Can you work these out from the model? Positions are in its coordinate system, mm. Face numbers are marked on the shaded views. Coordinates: 2 decimals unless noted, no trailing zeros. Write each loop counter-clockwise with the first axis right and the second up, starting at its lowest first coordinate (ties: lowest second). Pieces come first, ordered by that corner, then holes. Notation, with made-up numbers: (79, 38.25) - (130, 38.25) arc R29 cw to (130, 71.25) - close; hole circle Ø4 at (73.5, 87). An arc over 180 degrees is marked (long way). Write each question's results on one line, items separated by ' | '. Start each with the question number.
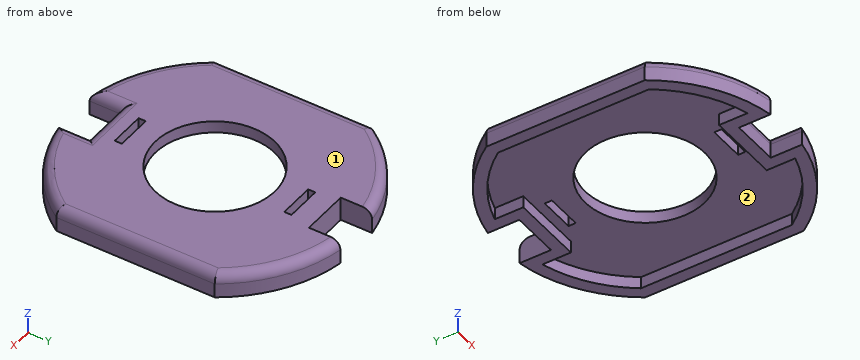
```python
from build123d import *

# Parameters (mm, degrees)
BOSS_EXTRUDE1_DEPTH = 1
FILLET1_R           = 0.4
SHELL1_DEPTH        = 0.5
SKETCH3_R           = 2.5
CUT_EXTRUDE1_DEPTH  = 1
CUT_EXTRUDE2_REACH  = 9.81
SKETCH4_W           = 1.5
SKETCH4_H           = 0.3


# Read off the part's stored shape, not the designer's step: Shell1
with BuildPart() as part:
    # Sketch2 → Boss-Extrude1 (new body)
    with BuildSketch(Plane.XY):
        with BuildLine():
            Line((-5, -3.31662479), (-5, 3.31662479))
            ThreePointArc((-5, 3.31662479), (-3.269448205, 5.030974899), (-1, 5.916079783))
            Line((-1, 5.916079783), (-1, 4.6))
            Line((-1, 4.6), (1, 4.6))
            Line((1, 4.6), (1, 5.916079783))
            ThreePointArc((1, 5.916079783), (3.269448205, 5.030974899), (5, 3.31662479))
            Line((5, 3.31662479), (5, -3.31662479))
            ThreePointArc((5, -3.31662479), (3.269448205, -5.030974899), (1, -5.916079783))
            Line((1, -5.916079783), (1, -4.6))
            Line((1, -4.6), (-1, -4.6))
            Line((-1, -4.6), (-1, -5.916079783))
            ThreePointArc((-1, -5.916079783), (-3.269448205, -5.030974899), (-5, -3.31662479))
        make_face()
    extrude(amount=BOSS_EXTRUDE1_DEPTH)

    # Fillet1
    fillet1_edges = [part.edges().sort_by_distance(p)[0] for p in [
        (3.269448205, 5.030974899, 1),
        (5, 0, 1),
        (3.269448205, -5.030974899, 1),
        (1, -5.258039892, 1),
        (0, -4.6, 1),
        (-1, -5.258039892, 1),
        (-3.269448205, -5.030974899, 1),
        (-5, 0, 1),
        (-3.269448205, 5.030974899, 1),
    ]]
    fillet(fillet1_edges, radius=FILLET1_R)

    # Shell1 outline → Shell1 (cut)
    with BuildSketch(Plane.XY):
        with BuildLine():
            ThreePointArc((1.5, -5.291502622), (3.183300133, -4.485153316), (4.5, -3.16227766))
            Line((4.5, -3.16227766), (4.5, 3.16227766))
            ThreePointArc((4.5, 3.16227766), (3.183300133, 4.485153316), (1.5, 5.291502622))
            Line((1.5, 5.291502622), (1.5, 4.1))
            Line((1.5, 4.1), (-1.5, 4.1))
            Line((-1.5, 4.1), (-1.5, 5.291502622))
            ThreePointArc((-1.5, 5.291502622), (-3.183300133, 4.485153316), (-4.5, 3.16227766))
            Line((-4.5, 3.16227766), (-4.5, -3.16227766))
            ThreePointArc((-4.5, -3.16227766), (-3.183300133, -4.485153316), (-1.5, -5.291502622))
            Line((-1.5, -5.291502622), (-1.5, -4.1))
            Line((-1.5, -4.1), (1.5, -4.1))
            Line((1.5, -4.1), (1.5, -5.291502622))
        make_face()
    extrude(amount=SHELL1_DEPTH, mode=Mode.SUBTRACT)

    # Sketch3 → Cut-Extrude1 (cut)
    with BuildSketch(Plane.XY.offset(1)):
        Circle(SKETCH3_R)
    extrude(amount=-CUT_EXTRUDE1_DEPTH, mode=Mode.SUBTRACT)

    # Sketch4 → Cut-Extrude2 (cut, up to next)
    with BuildSketch(Plane.XY.offset(1), mode=Mode.PRIVATE) as cut_extrude2_sk1:
        with Locations((0, 3.55)):
            Rectangle(SKETCH4_W, SKETCH4_H)
    cut_extrude2_tool1 = extrude(cut_extrude2_sk1.sketch, amount=-CUT_EXTRUDE2_REACH, mode=Mode.PRIVATE) & part.part
    # Sketch4 → Cut-Extrude2 (cut, up to next)
    with BuildSketch(Plane.XY.offset(1), mode=Mode.PRIVATE) as cut_extrude2_sk2:
        with Locations((0, -3.55)):
            Rectangle(SKETCH4_W, SKETCH4_H)
    cut_extrude2_tool2 = extrude(cut_extrude2_sk2.sketch, amount=-CUT_EXTRUDE2_REACH, mode=Mode.PRIVATE) & part.part
    add(cut_extrude2_tool1.solids().sort_by_distance((0, 3.55, 1))[0], mode=Mode.SUBTRACT)
    add(cut_extrude2_tool2.solids().sort_by_distance((0, -3.55, 1))[0], mode=Mode.SUBTRACT)


solid = part.part
```
Q1. I'm going to push flat-ended pins straight in: pin 1 Ø0.6 at (x, z) = (0.5, 0) entering from +Y; pin 2 Ø0.6 at (x, z) = (0.5, 1) entering from -Y. Where does each tip first touch, or does it pass through?
Q2. I need wall thicknesses on line 1 along X through (y, z) = (-2.25, 0.45); line 2 along X through (y, z) = (-4.75, 0.4); line 3 along Y through (x, z) = (0, 0.75). Which ranges of each line are inside material? Lowest first, please. Write a range as from..to.
Q3. If we section it at B-B (z = 0.15): Please give me the cut outline in (x, y), then the cut area to 3 significant figures.
Q4. If we section it at D-D (y = 2): Please give me the cut outline in (x, z), then the cut area to 3 significant figures.
Q5. Thinking about a two-plate mould opening in X: for the marked faces 1 and 2, which applies, pulls with the +X half, pulls with the -X half, needs draft (parallel to the pull), parting line crosses it, or undercut?
Q6. If we section it at A-A (y = 0): Please give me the cut outline in (x, z).
Q7. If we section it at C-C (x = 0): Please give me the cut outline in (y, z).
Answer list:
1) pin 1: stops at y = 4.6 | pin 2: stops at y = -4.59
2) line 1: x = -5..-4.5, 4.5..5 | line 2: x = -3.67..-2.77, -1.5..-1, 1..1.5, 2.77..3.67 | line 3: y = -4.57..-3.7, -3.4..-2.5, 2.5..3.4, 3.7..4.6
3) outline: (-5, -3.32) arc R6 ccw to (-1, -5.92) - (-1, -4.6) - (1, -4.6) - (1, -5.92) arc R6 ccw to (5, -3.32) - (5, 3.32) arc R6 ccw to (1, 5.92) - (1, 4.6) - (-1, 4.6) - (-1, 5.92) arc R6 ccw to (-5, 3.32) - close; hole (-4.5, -3.16) arc R5.5 ccw to (-1.5, -5.29) - (-1.5, -4.1) - (1.5, -4.1) - (1.5, -5.29) arc R5.5 ccw to (4.5, -3.16) - (4.5, 3.16) arc R5.5 ccw to (1.5, 5.29) - (1.5, 4.1) - (-1.5, 4.1) - (-1.5, 5.29) arc R5.5 ccw to (-4.5, 3.16) - close | area: 20.2 mm2
4) outline: (-5, 0) - (-4.5, 0) - (-4.5, 0.5) - (-1.5, 0.5) - (-1.5, 1) - (-4.6, 1) arc R0.4 ccw to (-5, 0.6) - close; (1.5, 0.5) - (4.5, 0.5) - (4.5, 0) - (5, 0) - (5, 0.6) arc R0.4 ccw to (4.6, 1) - (1.5, 1) - close | area: 3.93 mm2
5) face 1: needs draft | face 2: undercut
6) outline: (-5, 0) - (-4.5, 0) - (-4.5, 0.5) - (-2.5, 0.5) - (-2.5, 1) - (-4.6, 1) arc R0.4 ccw to (-5, 0.6) - close; (2.5, 0.5) - (4.5, 0.5) - (4.5, 0) - (5, 0) - (5, 0.6) arc R0.4 ccw to (4.6, 1) - (2.5, 1) - close
7) outline: (-4.6, 0) - (-4.1, 0) - (-4.1, 0.5) - (-3.7, 0.5) - (-3.7, 1) - (-4.2, 1) arc R0.4 ccw to (-4.6, 0.6) - close; (-3.4, 0.5) - (-2.5, 0.5) - (-2.5, 1) - (-3.4, 1) - close; (2.5, 0.5) - (3.4, 0.5) - (3.4, 1) - (2.5, 1) - close; (3.7, 0.5) - (4.1, 0.5) - (4.1, 0) - (4.6, 0) - (4.6, 1) - (3.7, 1) - close
